Can you work these out from the model? Positions are in its coordinate system, mm. Face numbers are marked on the shaded views. A direction names the side the tool comes from. Coordinates: 2 decimals unless noted, no trailing zeros. Order: outer loops, then holes, each group sorted by start corner. A loop starts at its lowest first (then second) coordinate and runs counter-clockwise, first axis right, second up. Notation, with made-up numbers: (-11, 84) - (18, 84) arc R8 cw to (18, 96) - close; hole circle Ø11 at (83, -0.5). An arc over 180 degrees is marked (long way). Use a Markdown table: item, result. Add a question column.
(1) If I drill on L1, parallel to X at y = 38.5, z = 0; L2, parallel to Y at x = 54.5, z = -40.5; L3, parallel to X at y = 107.5, z = 8, over which ranges is the centre line in solid material (lowest first)? Write a range as [from, to].
(2) On a 3-axis mill with a long thin cutter (end or side, diameter ignored), from which of +Z, -Z, +X, -X, +Y, -Y can I reach the whole of each face in a straight line? I mean the marked faces 4 and 5. Say none if no direction works.
(3) We'd pull the mould along Y, two halves only. Please class the marked faces 1, 2 and 3: pulls with the +Y half, pulls with the -Y half, needs draft (parallel to the pull), parting line crosses it, or undercut.
(4) For pin 1 Ø11 at (x, y) = (-1, -52) entering from +Z; pin 2 Ø12 at (x, y) = (15, 4.5) entering from +Z; pin 3 Ø5 at (y, z) = (-50, -28) entering from -X, each with a flat end and sliding along its axis, tell me the tip position at first contact or that it passes through.
(5) I want a section at A-A (y = -38). List the corners of the cut face in (x, z) for me, and give its area (3 significant figures).
```python
from build123d import *

# Parameters (mm, degrees)
SKETCH1_W               = 30
SKETCH1_H               = 30
SKETCH1_R               = 1.63
BOSS_EXTRUDE1_DEPTH     = 2.5
SKETCH2_R               = 12.5
CUT_EXTRUDE1_DEPTH      = 22.360009363
BOSS_EXTRUDE2_START     = 40
SKETCH3_R               = 13.5
SKETCH3_R_2             = 12.5
BOSS_EXTRUDE2_DEPTH     = 40
BOSS_EXTRUDE3_START     = -5
SKETCH4_R               = 15.5
BOSS_EXTRUDE3_DEPTH     = 1
LPATTERN1_COUNT         = 7
LPATTERN1_PITCH         = 5
CUT_EXTRUDE2_DEPTH      = 11
CUT_EXTRUDE2_DEPTH_BACK = 45.30293444
SKETCH5_R               = 12.5
SCALE1_SCALE            = 4
SKETCH8_W               = 120
SKETCH8_H               = 120
BOSS_EXTRUDE5_DEPTH     = 10
SKETCH9_R               = 6.8
CUT_EXTRUDE3_DEPTH      = 10
CUT_EXTRUDE4_REACH      = 202.22
SKETCH10_R              = 50


with BuildPart() as part:
    # Sketch1 → Boss-Extrude1 (new body)
    with BuildSketch(Plane(origin=(0, 0, 0), x_dir=(1, 0, 0), z_dir=(0, 1, 0))):
        Rectangle(SKETCH1_W, SKETCH1_H)
        with Locations(Location((-12.5, 12.5, 0), (0, 0, 270))):
            Circle(SKETCH1_R, mode=Mode.SUBTRACT)
        with Locations(Location((12.5, 12.5, 0), (0, 0, 270))):
            Circle(SKETCH1_R, mode=Mode.SUBTRACT)
        with Locations(Location((12.5, -12.5, 0), (0, 0, 270))):
            Circle(SKETCH1_R, mode=Mode.SUBTRACT)
        with Locations(Location((-12.5, -12.5, 0), (0, 0, 270))):
            Circle(SKETCH1_R, mode=Mode.SUBTRACT)
    extrude(amount=BOSS_EXTRUDE1_DEPTH)

    # Sketch2 → Cut-Extrude1 (cut, through all)
    with BuildSketch(Plane(origin=(0, 2.5, 0), x_dir=(1, 0, 0), z_dir=(0, 1, 0))):
        with Locations(Location((0, 0, 0), (0, 0, 270))):
            Circle(SKETCH2_R)
    extrude(amount=-CUT_EXTRUDE1_DEPTH, mode=Mode.SUBTRACT)

    # Sketch3 → Boss-Extrude2 (add)
    with BuildSketch(Plane(origin=(0, 2.5, 0), x_dir=(1, 0, 0), z_dir=(0, 1, 0)).offset(BOSS_EXTRUDE2_START)):
        with Locations(Location((0, 0, 0), (0, 0, 270))):
            Circle(SKETCH3_R)
        with Locations(Location((0, 0, 0), (0, 0, 270))):
            Circle(SKETCH3_R_2, mode=Mode.SUBTRACT)
    extrude(amount=-BOSS_EXTRUDE2_DEPTH)

    # Sketch4 → Boss-Extrude3 (add)
    with BuildSketch(Plane(origin=(0, 42.5, 0), x_dir=(1, 0, 0), z_dir=(0, 1, 0)).offset(BOSS_EXTRUDE3_START)):
        with Locations(Location((0, 0, 0), (0, 0, 270))):
            Circle(SKETCH4_R)
    boss_extrude3 = extrude(amount=BOSS_EXTRUDE3_DEPTH)

    # LPattern1: Boss-Extrude3 ×7
    with Locations(*[(0, -i * LPATTERN1_PITCH, 0) for i in range(1, LPATTERN1_COUNT)]):
        add(boss_extrude3)

    # Sketch5 → Cut-Extrude2 (cut, two sides: drawn at the far end of the back side and taken through both)
    with BuildSketch(Plane(origin=(0, 38.5, 0), x_dir=(1, 0, 0), z_dir=(0, 1, 0)).offset(-CUT_EXTRUDE2_DEPTH_BACK)):
        with Locations(Location((0, 0, 0), (0, 0, 270))):
            Circle(SKETCH5_R)
    extrude(amount=CUT_EXTRUDE2_DEPTH + CUT_EXTRUDE2_DEPTH_BACK, mode=Mode.SUBTRACT)


with BuildPart() as part_1:
    # Scale1: scaled about (0, 18.975181949, 0)
    add(part.part.scale(SCALE1_SCALE).moved(Location((0, -56.925545847, 0))))

    # Sketch8 → Boss-Extrude5 (add)
    with BuildSketch(Plane(origin=(0, 113.074454153, 0), x_dir=(1, 0, 0), z_dir=(0, 1, 0))):
        Rectangle(SKETCH8_W, SKETCH8_H)
    extrude(amount=BOSS_EXTRUDE5_DEPTH)

    # Sketch9 → Cut-Extrude3 (cut)
    with BuildSketch(Plane(origin=(0, 123.074454153, 0), x_dir=(1, 0, 0), z_dir=(0, 1, 0))):
        with Locations(Location((50, -50, 0), (0, 0, 270))):
            Circle(SKETCH9_R)
        with Locations(Location((-50, -50, 0), (0, 0, 90))):
            Circle(SKETCH9_R)
        with Locations(Location((-50, 50, 0), (0, 0, 270))):
            Circle(SKETCH9_R)
        with Locations(Location((50, 50, 0), (0, 0, 90))):
            Circle(SKETCH9_R)
    extrude(amount=-CUT_EXTRUDE3_DEPTH, mode=Mode.SUBTRACT)

    # Sketch10 → Cut-Extrude4 (cut, up to next)
    with BuildSketch(Plane.XZ.offset(56.925545847), mode=Mode.PRIVATE) as cut_extrude4_sk1:
        with Locations(Location((0, 0, 0), (0, 0, 90))):
            Circle(SKETCH10_R)
    cut_extrude4_tool1 = extrude(cut_extrude4_sk1.sketch, amount=-CUT_EXTRUDE4_REACH, mode=Mode.PRIVATE) & part_1.part
    add(cut_extrude4_tool1.solids().sort_by_distance((0, -56.925546, 0))[0], mode=Mode.SUBTRACT)


solid = part_1.part
```
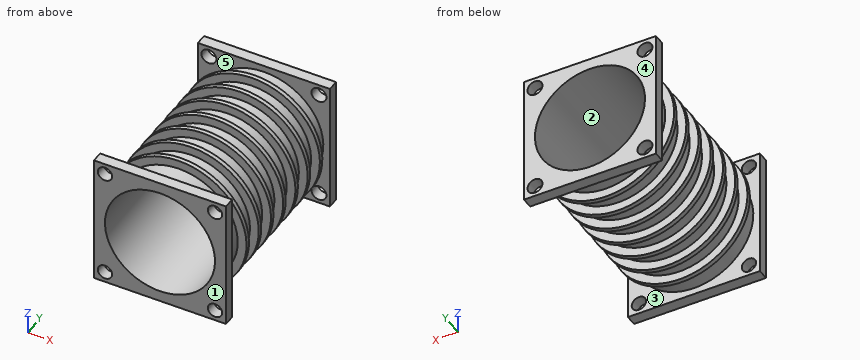
Answers follow:
| question | item | result |
|---|---|---|
| 1 | L1 | x = [-54, -50], [50, 54] |
| 1 | L2 | y = [-56.93, -46.93], [113.07, 123.07] |
| 1 | L3 | x = [-53.4, -49.36], [49.36, 53.4] |
| 2 | face 4 | +Z, -Z, +X, -X, +Y |
| 2 | face 5 | none |
| 3 | face 1 | pulls with the -Y half |
| 3 | face 2 | needs draft |
| 3 | face 3 | undercut |
| 4 | pin 1 | stops at z = 60 |
| 4 | pin 2 | stops at z = 53.24 |
| 4 | pin 3 | stops at x = -60 |
| 5 | outline | circle Ø108 at (0, 0); hole circle Ø100 at (0, 0) |
| 5 | area | 1,310 mm² |
